from build123d import *

# Parameters (mm, degrees)
SKETCH1_W           = 135
SKETCH1_H           = 15
BOSS_EXTRUDE1_DEPTH = 7.5
CUT_EXTRUDE1_REACH  = 74.715
CUT_EXTRUDE2_REACH  = 76.246
SKETCH4_W           = 27.679491924
SKETCH4_H           = 5
BOSS_EXTRUDE2_START = -15
SKETCH5_R           = 2.5
BOSS_EXTRUDE2_DEPTH = 15


with BuildPart() as part:
    # Sketch1 → Boss-Extrude1 (new, symmetric)
    with BuildSketch(Plane.XY):
        Rectangle(SKETCH1_W, SKETCH1_H)
        Polygon((22.5, -7.5), (-22.5, -7.5), (-13.839745962, -22.5), (13.839745962, -22.5), align=None)
    extrude(amount=BOSS_EXTRUDE1_DEPTH, both=True)

    # Sketch2 → Cut-Extrude1 (cut, up to next)
    with BuildSketch(Plane.XY.offset(7.5), mode=Mode.PRIVATE) as cut_extrude1_sk1:
        with BuildLine():
            Line((2.5, 2.5), (2.5, -17.5))
            ThreePointArc((2.5, -17.5), (0, -20), (-2.5, -17.5))
            Line((-2.5, -17.5), (-2.5, 2.5))
            ThreePointArc((-2.5, 2.5), (0, 5), (2.5, 2.5))
        make_face()
    cut_extrude1_tool1 = extrude(cut_extrude1_sk1.sketch, amount=-CUT_EXTRUDE1_REACH, mode=Mode.PRIVATE) & part.part
    # Sketch2 → Cut-Extrude1 (cut, up to next)
    with BuildSketch(Plane.XY.offset(7.5), mode=Mode.PRIVATE) as cut_extrude1_sk2:
        with BuildLine():
            Line((10.1, -4.903635329), (10.1, -24.903635329))
            ThreePointArc((10.1, -24.903635329), (8, -27.003635329), (5.9, -24.903635329))
            Line((5.9, -24.903635329), (5.9, -4.903635329))
            ThreePointArc((5.9, -4.903635329), (8, -2.803635329), (10.1, -4.903635329))
        make_face()
    cut_extrude1_tool2 = extrude(cut_extrude1_sk2.sketch, amount=-CUT_EXTRUDE1_REACH, mode=Mode.PRIVATE) & part.part
    # Sketch2 → Cut-Extrude1 (cut, up to next)
    with BuildSketch(Plane.XY.offset(7.5), mode=Mode.PRIVATE) as cut_extrude1_sk3:
        with BuildLine():
            Line((-5.9, -4.903635329), (-5.9, -24.903635329))
            ThreePointArc((-5.9, -24.903635329), (-8, -27.003635329), (-10.1, -24.903635329))
            Line((-10.1, -24.903635329), (-10.1, -4.903635329))
            ThreePointArc((-10.1, -4.903635329), (-8, -2.803635329), (-5.9, -4.903635329))
        make_face()
    cut_extrude1_tool3 = extrude(cut_extrude1_sk3.sketch, amount=-CUT_EXTRUDE1_REACH, mode=Mode.PRIVATE) & part.part
    add(cut_extrude1_tool1.solids().sort_by_distance((0, -7.5, 7.5))[0], mode=Mode.SUBTRACT)
    add(cut_extrude1_tool2.solids().sort_by_distance((8, -14.903635, 7.5))[0], mode=Mode.SUBTRACT)
    add(cut_extrude1_tool3.solids().sort_by_distance((-8, -14.903635, 7.5))[0], mode=Mode.SUBTRACT)

    # Sketch4 → Cut-Extrude2 (cut, up to next)
    with BuildSketch(Plane.XZ.offset(22.5), mode=Mode.PRIVATE) as cut_extrude2_sk1:
        with Locations((0, 5)):
            Rectangle(SKETCH4_W, SKETCH4_H)
    cut_extrude2_tool1 = extrude(cut_extrude2_sk1.sketch, amount=-CUT_EXTRUDE2_REACH, mode=Mode.PRIVATE) & part.part
    # Sketch4 → Cut-Extrude2 (cut, up to next)
    with BuildSketch(Plane.XZ.offset(22.5), mode=Mode.PRIVATE) as cut_extrude2_sk2:
        with Locations((0, -5)):
            Rectangle(SKETCH4_W, SKETCH4_H)
    cut_extrude2_tool2 = extrude(cut_extrude2_sk2.sketch, amount=-CUT_EXTRUDE2_REACH, mode=Mode.PRIVATE) & part.part
    add(cut_extrude2_tool1.solids().sort_by_distance((0, -22.5, 5))[0], mode=Mode.SUBTRACT)
    add(cut_extrude2_tool2.solids().sort_by_distance((0, -22.5, -5))[0], mode=Mode.SUBTRACT)

    # Sketch5 → Boss-Extrude2 (add)
    with BuildSketch(Plane(origin=(0, 7.5, 0), x_dir=(1, 0, 0), z_dir=(0, 1, 0)).offset(BOSS_EXTRUDE2_START)):
        with Locations(Location((61.994193156, 0, 0), (0, 0, 270))):
            Circle(SKETCH5_R)
        with Locations(Location((-61.994193156, 0, 0), (0, 0, 270))):
            Circle(SKETCH5_R)
    extrude(amount=-BOSS_EXTRUDE2_DEPTH)


solid = part.part
CAD build for the part. Positions are in the model's coordinates, mm. A direction names the side the tool comes from. Round coordinates to 2 decimals unless told otherwise and drop trailing zeros. Order: outer loops, then holes, each group sorted by start corner. A loop starts at its lowest first (then second) coordinate and runs counter-clockwise, first axis right, second up. Notation, with made-up numbers: (-35.5, -5) - (-31.5, -5) arc R24 ccw to (-31.5, 21) - close; hole circle Ø5 at (1, 50.5). An arc over 180 degrees is marked (long way). Return JSON: item names as keys, results as strings.
(1) Cut at A-A (z = 3.75). Give the cut face in (x, y).
Answer key:
{"outline": "(-67.5, -7.5) - (-22.5, -7.5) - (-13.84, -22.5) - (-13.84, 7.5) - (-67.5, 7.5) - close; (13.84, -22.5) - (22.5, -7.5) - (67.5, -7.5) - (67.5, 7.5) - (13.84, 7.5) - close"}
(2) Cut at C-C (x = 29). Give the cut face in (y, z), then the cut area to 3 significant figures.
Answer key:
{"outline": "(-7.5, -7.5) - (7.5, -7.5) - (7.5, 7.5) - (-7.5, 7.5) - close", "area": "225 mm^2"}
(3) Pin check, flat tips, straight feed: pin 1 Ø1.5 at (y, z) = (-17.5, 3.5) entering from +X; pin 2 Ø7.5 at (x, z) = (-44.5, -2.5) entering from -Y; pin 3 Ø1.5 at (y, z) = (-17.5, -1) entering from +X. Stop position of each tip, or through.
Answer key:
{"pin 1": "stops at x = 17.16", "pin 2": "stops at y = -7.5", "pin 3": "stops at x = 64.48"}
(4) Wall check: probe 1 along X at (y, z) = (-7, 2.25); probe 2 along X at (y, z) = (4.75, -2.75); probe 3 along X at (y, z) = (-3.25, 0.5). Give the ranges that are in metal, low to high. Write a range as from..to.
Answer key:
{"probe 1": "x = -67.5..-10.1, -5.9..-2.5, 2.5..5.9, 10.1..67.5", "probe 2": "x = -67.5..-13.84, 13.84..67.5", "probe 3": "x = -67.5..-9.29, -6.71..-2.5, 2.5..6.71, 9.29..67.5"}
(5) Tool access for faces 1 (the face through (-10.1, -14, 0)), 2 (the face through (-13.84, -8, -5)), 3 (the face through (-59.515, -14.895, -0.325)), 4 (the face through (13.84, -8, 5)), 5 (the face through (0, 5, 0)): list every direction of +Z, -Z, +X, -X, +Y, -Y with a clear straight run to the whole face (end or side of a thin tool).
Answer key:
{"face 1": "+Z, -Z, -Y", "face 2": "-Z, +Y, -Y", "face 3": "-Y", "face 4": "+Z, +Y, -Y", "face 5": "+Z, -Z"}
(6) Cut at B-B (x = 0). Give the cut face in (y, z).
Answer key:
{"outline": "(-22.5, -2.5) - (-20, -2.5) - (-20, 2.5) - (-22.5, 2.5) - close; (5, -2.5) - (7.5, -2.5) - (7.5, 2.5) - (5, 2.5) - close"}
(7) Pull direction Y, two halves, no side cores. Call faces 6 (the face through (2.5, -7, 0)), 7 (the face through (-67.5, 0, 0)), 8 (the face through (-18.23, -14.895, 0.105)): +Y half, -Y half, draft (parallel to the pull), parting line (faces both ways), or undercut.
Answer key:
{"face 6": "undercut", "face 7": "draft", "face 8": "-Y half"}
